The listing builds one solid part. Answer for the finished solid, in the listing's coordinates (mm). A direction names the side the tool comes from. Give positions to 0.01 mm unless a question says otherwise; leave off trailing zeros. Write each loop counter-clockwise with the first axis right and the second up, starting at its lowest first coordinate (ties: lowest second). Pieces come first, ordered by that corner, then holes. Notation, with made-up numbers: (-11, 55) - (34, 55) arc R21 cw to (34, 81) - close; hole circle Ø5 at (19.25, 12.5). An arc over 180 degrees is marked (long way). One line per question, with ' | ' between items. Start each with the question number.
1. The mould has two halves that part along Z. Classify faces 1 (the face through (-3.15, 1.774, 4.056)), 2 (the face through (2, 0, -5)), 3 (the face through (7.493, 1.771, 0.33)): +Z half, -Z half, draft (parallel to the pull), parting line (faces both ways), or undercut.
2. A cutting plane is placed at B-B (x = 0). Determine the outline of the cut face in (y, z).
3. Given P1, Ø1, axis at y = 0.5, z = 4, coming from the +X side; P2, Ø2.5, axis at x = -2, z = 1, coming from the -Y side; P3, Ø3.5, axis at x = 0, z = 0, coming from the -Y side; P4, Ø1, axis at x = -3, y = 2.5, coming from the -Z side, each flat-ended and moving along its own axis, determine where each tip first touches the part or whether it passes through.
4. A cutting plane is placed at C-C (y = 0.9). Determine the outline of the cut face in (x, z).
5. Find the intervals of material crossed by L1, parallel to Z at x = 0, y = 2.8; L2, parallel to Z at x = 2.25, y = 2.75; L3, parallel to X at y = 0.7, z = -3.5, in increasing order. Write a range as from..to.
6. For faces 4 (the face through (-3.15, 1.774, -6.336)), 5 (the face through (0.991, 1.113, -4.463)), determine the directions among +Z, -Z, +X, -X, +Y, -Y from which every point of the face is accessible in a straight line to the end or side of a thin tool.
7. A cutting plane is placed at A-A (z = 0). State how many separate pieces and enclosed holes the cut face has, then the cut area to 3 significant figures.
```python
from build123d import *

# Parameters (mm, degrees)
SKETCH2_R          = 1.15
CUT_EXTRUDE1_DEPTH = 10
FILLET3_R          = 0.25
FILLET4_R          = 0.25
FILLET5_R          = 0.25


with BuildPart() as part:
    # Sketch1 → Revolve1 (revolve)
    with BuildSketch(Plane.XY):
        Polygon((-4.572, 0), (-7.5, 0), (-7.5, 3.5), (-3.0734, 3.5), (-3.0734, 2), (-4.572, 2), align=None)
    revolve(axis=Axis((0, 0, 0), (0, 1, 0)))

    # Sketch2 → Cut-Extrude1 (cut)
    with BuildSketch(Plane(origin=(0, 3.5, 0), x_dir=(1, 0, 0), z_dir=(0, 1, 0))):
        with Locations((6, 0)):
            Circle(SKETCH2_R)
        with Locations((-3, -5.196152423)):
            Circle(SKETCH2_R)
        with Locations((-3, 5.196152423)):
            Circle(SKETCH2_R)
    extrude(amount=-CUT_EXTRUDE1_DEPTH, mode=Mode.SUBTRACT)

    # Fillet3
    fillet3_edges = [part.edges().sort_by_distance(p)[0] for p in [
        (3.0734, 3.5, 0),
    ]]
    fillet(fillet3_edges, radius=FILLET3_R)

    # Fillet4
    fillet4_edges = [part.edges().sort_by_distance(p)[0] for p in [
        (7.5, 3.5, 0),
    ]]
    fillet(fillet4_edges, radius=FILLET4_R)

    # Fillet5
    fillet5_edges = [part.edges().sort_by_distance(p)[0] for p in [
        (7.5, 0, 0),
        (4.572, 0, 0),
    ]]
    fillet(fillet5_edges, radius=FILLET5_R)


solid = part.part
```
Determined:
1) face 1: undercut | face 2: draft | face 3: parting line
2) outline: (0, -7.25) arc R0.25 ccw to (0.25, -7.5) - (3.25, -7.5) arc R0.25 ccw to (3.5, -7.25) - (3.5, -3.32) arc R0.25 ccw to (3.25, -3.07) - (2, -3.07) - (2, -4.57) - (0.25, -4.57) arc R0.25 ccw to (0, -4.82) - close; (0, 4.82) arc R0.25 ccw to (0.25, 4.57) - (2, 4.57) - (2, 3.07) - (3.25, 3.07) arc R0.25 ccw to (3.5, 3.32) - (3.5, 7.25) arc R0.25 ccw to (3.25, 7.5) - (0.25, 7.5) arc R0.25 ccw to (0, 7.25) - close
3) P1: x = 6.63 | P2: y = 2 | P3: through | P4: z = -7.07
4) outline: circle Ø15 at (0, 0); hole circle Ø9.14 at (0, 0); hole circle Ø2.3 at (-3, -5.2); hole circle Ø2.3 at (-3, 5.2); hole circle Ø2.3 at (6, 0)
5) L1: -7.5..-3.07, 3.07..7.5 | L2: -7.15..-2.09, 2.09..7.15 | L3: -6.63..-2.94, 2.94..6.63
6) face 4: +Y, -Y | face 5: -Y
7) separate pieces: 3 | enclosed holes: 0 | area: 16.8 mm2
